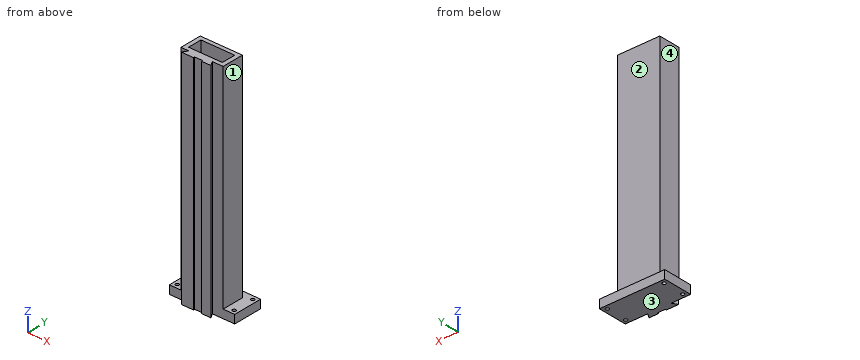
from build123d import *

# Parameters (mm, degrees)
SKETCH002_W  = 80
SKETCH002_H  = 33.5
PAD_DEPTH    = 505
SKETCH001_R  = 4
PAD001_DEPTH = 20


with BuildPart() as part:
    # Sketch002 → Pad (new body)
    with BuildSketch(Plane.XY):
        Polygon((-50, 0), (50, 0), (50, -52), (24.5, -52), (31.428203, -64), (9.65, -64), (9.65, -61), (-9.65, -61), (-9.65, -64), (-38.428203, -64), (-31.5, -52), (-50, -52), align=None)
        with Locations((0, -26)):
            Rectangle(SKETCH002_W, SKETCH002_H, mode=Mode.SUBTRACT)
    extrude(amount=PAD_DEPTH)

    # Sketch001 → Pad001 (new body)
    with BuildSketch(Plane(origin=(0, 0, 0), x_dir=(1, 0, 0), z_dir=(0, 0, -1))):
        Polygon((77.5, 52), (77.5, -18), (-77.5, -18), (-77.5, 52), (-31.5, 52), (-38.428203, 64), (-9.65, 64), (-9.65, 61), (9.65, 61), (9.65, 64), (31.428203, 64), (24.5, 52), align=None)
        with Locations((-67.5, 42)):
            Circle(SKETCH001_R, mode=Mode.SUBTRACT)
        with Locations((-67.5, -8)):
            Circle(SKETCH001_R, mode=Mode.SUBTRACT)
        with Locations((67.5, 42)):
            Circle(SKETCH001_R, mode=Mode.SUBTRACT)
        with Locations((67.5, -8)):
            Circle(SKETCH001_R, mode=Mode.SUBTRACT)
    extrude(amount=PAD001_DEPTH)


solid = part.part
Geometry: final body of the model. Coordinates: model frame, mm. Face numbers are marked on the shaded views. A direction names the side the tool comes from. Give positions to 0.01 mm unless a question says otherwise; leave off trailing zeros. Loops run counter-clockwise (first coordinate to the right, second up) from the corner with the lowest first, then second, coordinate; pieces in that order, holes last. Notation, with made-up numbers: (20.5, 23) -> (36.5, 23) arc R22 ccw to (36.5, 53) -> close; hole circle Ø8 at (86.25, 56). An arc over 180 degrees is marked (long way). Put each result on its own line as item: value.
1. Cut plane A-A (z = 45.5). Return the cut outline in (x, y), plus the area to 3 significant figures.
Taken from the geometry:
outline: (-50, -52) -> (-31.5, -52) -> (-38.43, -64) -> (-9.65, -64) -> (-9.65, -61) -> (9.65, -61) -> (9.65, -64) -> (31.43, -64) -> (24.5, -52) -> (50, -52) -> (50, 0) -> (-50, 0) -> close; hole (-40, -42.75) -> (40, -42.75) -> (40, -9.25) -> (-40, -9.25) -> close
area: 3,220 mm2
2. Cut plane B-B (x = 1). Return the cut outline in (y, z), plus the area to 3 significant figures.
Taken from the geometry:
outline: (-61, -20) -> (18, -20) -> (18, 0) -> (0, 0) -> (0, 505) -> (-9.25, 505) -> (-9.25, 0) -> (-42.75, 0) -> (-42.75, 505) -> (-61, 505) -> close
area: 15,500 mm2
3. Set-up query: the marked faces 1, 2, 3 and 4. Return all of +Z, -Z, +X, -X, +Y, -Y with unobstructed straight access to the full face (end or side cutting, diameter ignored); none if empty.
Taken from the geometry:
face 1: +Z, +X, +Y, -Y
face 2: +Z, +X, -X, +Y
face 3: -Z, +X, -X, +Y, -Y
face 4: +Z, -X, +Y, -Y
4. Ray query, line 1 along X through (y, z) = (8, -11.75); line 2 along Y through (x, z) = (-67.5, -9); line 3 along Y through (x, z) = (21.5, 287.5). Return the intervals inside material, ascending. Write a range as [from, to].
Taken from the geometry:
line 1: x = [-77.5, -71.5], [-63.5, 63.5], [71.5, 77.5]
line 2: y = [-52, -46], [-38, 4], [12, 18]
line 3: y = [-64, -42.75], [-9.25, 0]
5. Pin query (flat end, axial travel): P1, Ø1, axis at x = 10.5, z = 331.5, coming from the +Y side; P2, Ø17, axis at y = -18.5, z = 263, coming from the -X side; P3, Ø23, axis at x = -56.5, z = 293.5, coming from the -Y side; P4, Ø5, axis at x = -67.5, y = 8, coming from the +Z side. Return the tip coordinate at first contact, or that it passes through.
Taken from the geometry:
P1: stops at y = 0
P2: stops at x = -50
P3: stops at y = -52
P4: passes through
6. Cut plane C-C (y = -27.5). Return the cut outline in (x, z).
Taken from the geometry:
outline: (-77.5, -20) -> (77.5, -20) -> (77.5, 0) -> (50, 0) -> (50, 505) -> (40, 505) -> (40, 0) -> (-40, 0) -> (-40, 505) -> (-50, 505) -> (-50, 0) -> (-77.5, 0) -> close
